Autodesk Inventor part; units mm, degrees
ref_plane "YZ Plane" through (0, 0, 0) normal (1, 0, 0) x (0, 1, 0)
ref_plane "XZ Plane" through (0, 0, 0) normal (0, 1, 0) x (-1, 0, 0)
ref_plane "XY Plane" through (0, 0, 0) normal (0, 0, 1) x (1, 0, 0)
sketch "Sketch1" plane through (0, 0, 0) normal (0, 1, 0) x (-1, 0, 0)
  point P0 (0, 0)
sketch "Sketch2" plane through (0, 0, 0) normal (0, 1, 0) x (-1, 0, 0)
  line L0 (-6.55, 15.35) -> (6.55, 15.35)
  line L1 (6.55, 15.35) -> (6.55, -15.35)
  line L2 (6.55, -15.35) -> (-6.55, -15.35)
  line L3 (-6.55, -15.35) -> (-6.55, 15.35)
  line L4 (-6.55, 15.35) -> (6.55, -15.35) construction
  line L5 (6.55, 15.35) -> (-6.55, -15.35) construction
  line L6 (-9.525, 18.325) -> (9.525, 18.325)
  line L7 (9.525, 18.325) -> (9.525, -18.325)
  line L8 (9.525, -18.325) -> (-9.525, -18.325)
  line L9 (-9.525, -18.325) -> (-9.525, 18.325)
  line L10 (-9.525, 18.325) -> (9.525, -18.325) construction
  line L11 (9.525, 18.325) -> (-9.525, -18.325) construction
  point P0 (0, 0)
  dimension "d0" = 13.1
  dimension "d1" = 30.7
  dimension "d2" = 19.05
  dimension "d3" = 36.65
extrude "Extrusion1" add sketch "Sketch2" along normal blind 19.2
sketch "Sketch3" plane through (0, 19.2, 0) normal (0, 1, 0) x (1, 0, 0)
  line L0 (-9.525, -18.325) -> (9.525, -18.325)
  line L1 (9.525, -18.325) -> (9.525, 18.325)
  line L2 (9.525, 18.325) -> (-9.525, 18.325)
  line L3 (-9.525, 18.325) -> (-9.525, -18.325)
  point P0 (0, 0)
extrude "Extrusion2" add sketch "Sketch3" along normal blind 3
sketch "Sketch4" plane through (0, 22.2, 0) normal (0, 1, 0) x (1, 0, 0)
  line L0 (-6.55, -15.35) -> (-6.55, 15.35) construction
  line L1 (6.55, -15.35) -> (-6.55, -15.35) construction
  line L2 (-6.55, -15.35) -> (-6.55, 15.35) construction
  line L3 (-6.55, 15.35) -> (6.55, 15.35) construction
  line L4 (6.55, 15.35) -> (6.55, -15.35) construction
  line L5 (6.55, -15.35) -> (-6.55, 15.35) construction
  line L6 (-6.55, -15.35) -> (6.55, 15.35) construction
  line L7 (6.55, 15.35) -> (6.55, -15.35)
  line L8 (-6.55, -15.35) -> (6.55, -15.35)
  line L9 (6.55, -15.35) -> (6.55, -0.65)
  line L10 (6.55, -0.65) -> (-6.55, -0.65)
  line L11 (-6.55, -0.65) -> (-6.55, -15.35)
  point P0 (0, 0)
  point P1 (6.55, -15.35)
  dimension "d8" = 14.7
extrude "Extrusion3" cut sketch "Sketch4" against normal blind 5
sketch "Sketch6" plane through (9.525, 0, 18.325) normal (1, 0, 0) x (0, 0, -1)
  line L0 (0, 0) -> (36.65, 0) construction
  line L1 (0, 0) -> (11.925, 0) construction
  line L2 (11.925, 0) -> (11.925, 3) construction
  line L3 (11.925, 3) -> (0, 3) construction
  line L4 (0, 3) -> (0, 0) construction
  circle A0 centre (11.925, 3) radius 2.5
  line L5 (9.425, 3) -> (9.425, -0.2828)
  line L6 (14.425, 3) -> (14.425, 0)
  line L7 (9.425, 0) -> (14.425, 0)
  point P0 (18.325, 0)
  dimension "d16" = 11.925
  dimension "d17" = 3
  dimension "d18" = 5
extrude "Extrusion5" cut sketch "Sketch6" against normal through all
sketch "Sketch7" plane through (0, 22.2, 0) normal (0, 1, 0) x (1, 0, 0)
  line L0 (9.525, 18.325) -> (-9.525, 18.325)
  line L1 (-9.525, 18.325) -> (-9.525, -18.325)
  line L2 (9.525, 18.325) -> (-9.525, 18.325)
  line L3 (-9.525, 18.325) -> (-9.525, 1.325)
  line L4 (-9.525, 1.325) -> (9.525, 1.325)
  line L5 (9.525, 1.325) -> (9.525, 18.325)
  point P0 (0, 0)
  dimension "d21" = 17
extrude "Extrusion6" add sketch "Sketch7" along normal blind 11
sketch "Sketch8" plane through (9.525, 0, 18.325) normal (1, 0, 0) x (0, 0, -1)
  line L0 (19.65, 33.2) -> (36.65, 33.2) construction
  line L1 (28.15, 33.2) -> (28.15, 26.2) construction
  circle A0 centre (28.15, 26.2) radius 4
  point P0 (18.325, 0)
  dimension "d24" = 7
  dimension "d25" = 8
extrude "Extrusion7" cut sketch "Sketch8" against normal through all
sketch "Sketch9" plane through (9.525, 0, 18.325) normal (1, 0, 0) x (0, 0, -1)
  circle A0 centre (28.15, 26.2) radius 4 construction
  circle A1 centre (28.15, 26.2) radius 4 construction
  point P0 (18.325, 0)
hole "Hole1" at (9.525, 26.2, -9.825) direction (-1, 0, 0) diameter 8.566 depth 4
sketch "Sketch10" plane through (-9.525, 0, 18.325) normal (-1, 0, 0) x (0, 0, 1)
  circle A0 centre (-28.15, 26.2) radius 4 construction
  circle A1 centre (-28.15, 26.2) radius 4 construction
  point P0 (-18.325, 0)
hole "Hole2" at (-9.525, 26.2, -9.825) direction (1, 0, 0) diameter 8.566 depth 4
properties part number "ADAPTER_AOM-brimrose-watercooled-cover-2"
Verification items for the finished model (mm, model axes). A direction names the side the tool comes from. Give positions to 0.01 mm unless a question says otherwise; leave off trailing zeros. Write each loop counter-clockwise with the first axis right and the second up, starting at its lowest first coordinate (ties: lowest second). Pieces come first, ordered by that corner, then holes. Notation, with made-up numbers: M 26.25,80 L 74.25,80 A19 cw 74.25,94 Z; hole C 17,58.25 d7. An arc over 180 degrees is marked long. One line per question, with ' | ' between items.
1) Thickness scan on line 1 along X through (y, z) = (13.5, -2.5) (3 decimals); line 2 along Z through (x, y) = (-8.5, 26.2) (3 decimals); line 3 along Z through (x, y) = (-6, 14.5) (3 decimals). Record the ranges inside material, lowest first. Write a range as [from, to].
Result:
line 1: x = [-9.525, -6.55], [6.55, 9.525] | line 2: z = [-18.325, -14.108], [-5.542, -1.325] | line 3: z = [-18.325, -15.35], [15.35, 18.325]
2) Set-up check for faces 4 (the cylindrical face through (7.497, 21.953, -9.267)), 5 (the flat face through (0, 11, 15.35)), 6 (the flat face through (-9, 22.2, 8)), 7 (the flat face through (0, 9, -15.35)): record each of +Z, -Z, +X, -X, +Y, -Y from which the full face is reachable in a straight line by a thin tool's end or side.
Result:
face 4: +X | face 5: +Y, -Y | face 6: +Z, +X, -X, +Y | face 7: -Y
3) Section check C-C on z = 2.5. Enter the section's corners in (x, y) (3 decimals), plus the area to 3 significant figures.
Result:
outline: M -9.525,0 L -6.55,0 L -6.55,22.2 L -9.525,22.2 Z; M 6.55,0 L 9.525,0 L 9.525,22.2 L 6.55,22.2 Z | area: 132 mm2
4) Gauge pin test, flat ends, axial feed: pin 1 Ø4 at (x, z) = (-7.5, 8.5) entering from -Y; pin 2 Ø7.5 at (y, z) = (26.2, -9.825) entering from +X; pin 3 Ø4 at (x, z) = (-2.5, -6.5) entering from -Y; pin 4 Ø3.5 at (x, y) = (-4.5, 25.5) entering from +Z (3 decimals). Record the tip position at first contact, or that the pin passes through.
Result:
pin 1: stops at y = 0 | pin 2: passes through | pin 3: stops at y = 19.2 | pin 4: stops at z = -1.325
5) Section check A-A on x = 0.75. Enter the section's corners in (y, z) (3 decimals).
Result:
outline: M 0,-18.325 L 33.2,-18.325 L 33.2,-1.325 L 22.2,-1.325 L 22.2,0.65 L 19.2,0.65 L 19.2,-15.35 L 0,-15.35 Z; M 0,15.35 L 22.2,15.35 L 22.2,18.325 L 0,18.325 Z; hole C 26.2,-9.825 d8
6) Section check D-D on x = 8.5. Enter the section's corners in (y, z) (3 decimals), plus the area to 3 significant figures.
Result:
outline: M 0,-18.325 L 33.2,-18.325 L 33.2,-1.325 L 22.2,-1.325 L 22.2,18.325 L 0,18.325 L 0,8.9 L 3,8.9 A2.5 cw 3,3.9 L 0,3.9 Z; hole C 26.2,-9.825 d8.566 | area: 918 mm2
7) Mould release check, pull along Z, two halves, no side actions. Record for faces 1 (the flat face through (9.525, 13, 0)), 2 (the flat face through (0, 19.2, -7)), 3 (the flat face through (0, 16, -18.325)): released by +Z, released by -Z, zero draft, split by the parting line, or undercut.
Result:
face 1: zero draft | face 2: undercut | face 3: released by -Z
8) Section check B-B on y = 26.2. Enter the section's corners in (x, z) (3 decimals), plus the area to 3 significant figures.
Result:
outline: M -9.525,-18.325 L 9.525,-18.325 L 9.525,-14.108 L 5.525,-14.108 L 5.525,-13.825 L -5.525,-13.825 L -5.525,-14.108 L -9.525,-14.108 Z; M -9.525,-5.542 L -5.525,-5.542 L -5.525,-5.825 L 5.525,-5.825 L 5.525,-5.542 L 9.525,-5.542 L 9.525,-1.325 L -9.525,-1.325 Z | area: 167 mm2
